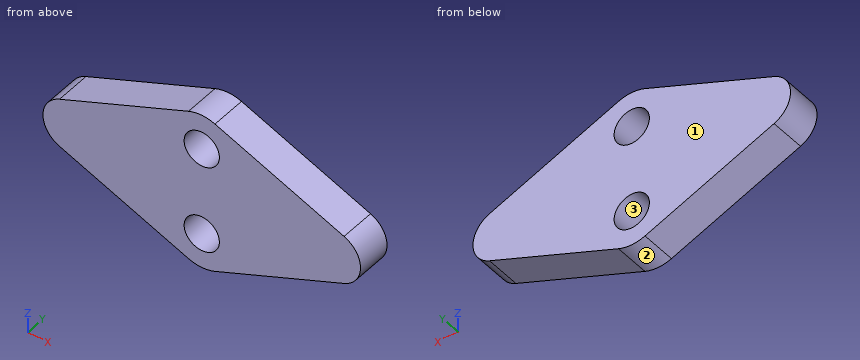
Autodesk Inventor part; units mm, degrees
ref_plane "YZ Plane" through (0, 0, 0) normal (1, 0, 0) x (0, 1, 0)
ref_plane "XZ Plane" through (0, 0, 0) normal (0, 1, 0) x (-1, 0, 0)
ref_plane "XY Plane" through (0, 0, 0) normal (0, 0, 1) x (1, 0, 0)
sketch "スケッチ1" plane through (0, 0, 0) normal (0, 1, 0) x (-1, 0, 0)
  circle A0 centre (7.5, 0) radius 1.5
  circle A1 centre (0, 2.5) radius 2
  circle A2 centre (0, -2.5) radius 2
  circle A3 centre (-7.5, 0) radius 1.5
  line L0 (7.5, 0) -> (-7.5, 0) construction
  line L1 (0, -2.5) -> (0, 2.5) construction
  line L2 (0.7512, 4.3536) -> (8.0634, 1.3902)
  line L3 (8.0634, -1.3902) -> (0.7512, -4.3536)
  line L4 (-0.7512, -4.3536) -> (-8.0634, -1.3902)
  line L5 (-8.0634, 1.3902) -> (-0.7512, 4.3536)
  point P0 (0, 0)
  point P1 (0, 0)
  dimension "d0" = 5
  dimension "d1" = 15
  dimension "d2" = 4
  dimension "d3" = 3
extrude "押し出し1" add sketch "スケッチ1" along normal blind 2
sketch "スケッチ2" plane through (0, 2, 0) normal (0, 1, 0) x (1, 0, 0)
  arc A0 (-0.7512, -4.3536) -> (0.7512, -4.3536) centre (0, -2.5) ccw
  arc A1 (0.7512, 4.3536) -> (-0.7512, 4.3536) centre (0, 2.5) ccw
  point P0 (0, 0)
hole "穴1" at (0, 2, 2.5) at (0, 2, -2.5) direction (0, -1, 0) diameter 2 end through all
properties part number "Band_Cap"
Build history of the part. All positions in model axes, mm. Face numbers are marked on the shaded views. Round coordinates to 2 decimals unless told otherwise and drop trailing zeros. Loops run counter-clockwise (first coordinate to the right, second up) from the corner with the lowest first, then second, coordinate; pieces in that order, holes last. Notation, with made-up numbers: (30.5, 59) -> (50.5, 59) arc R26 cw to (50.5, 74) -> close; hole circle Ø1 at (21, 30.5). An arc over 180 degrees is marked (long way). Use CSV: the item, a comma, the result in double quotes. Start each with the question number.
Q1. Saw through at A-A on z = -2.5. Give the cut face in (x, y), and give its area (3 significant figures).
Q2. Drill centre lines: L1, parallel to Z at x = 0.75, y = 0.9; L2, parallel to X at y = 0.65, z = -2.5; L3, parallel to X at y = 0.8, z = -1.75. Where is each one in solid material? Low to high.
Q3. Saw through at B-B on y = 1.3. Give the cut face in (x, z).
Q4. Saw through at C-C on x = -7.25. Give the cut face in (y, z).
Q5. Flat gauge pin, fed straight in: pin 1 Ø1.8 at (x, z) = (0, -2.5) entering from -Y. Where does the tip first touch, or does it go through?
Q6. Saw through at D-D on z = 3.25. Give the cut face in (x, y), and give its area (3 significant figures).
Q7. Mould opens along X. For the marked faces 1, 2 and 3 say: +X half, -X half, draft (parallel to the pull), parting line (faces both ways), or undercut.
Solutions:
1,outline,"(-5.32, 0) -> (-1, 0) -> (-1, 2) -> (-5.32, 2) -> close; (1, 0) -> (5.32, 0) -> (5.32, 2) -> (1, 2) -> close"
1,area,"17.3 mm^2"
2,L1,"z = -4.35 to -3.16, -1.84 to 1.84, 3.16 to 4.35"
2,L2,"x = -5.32 to -1, 1 to 5.32"
2,L3,"x = -7.18 to -0.66, 0.66 to 7.18"
3,outline,"(-8.06, -1.39) -> (-0.75, -4.35) arc R2 ccw to (0.75, -4.35) -> (8.06, -1.39) arc R1.5 ccw to (8.06, 1.39) -> (0.75, 4.35) arc R2 ccw to (-0.75, 4.35) -> (-8.06, 1.39) arc R1.5 ccw to start; hole circle Ø2 at (0, -2.5); hole circle Ø2 at (0, 2.5)"
4,outline,"(0, -1.72) -> (2, -1.72) -> (2, 1.72) -> (0, 1.72) -> close"
5,pin 1,"passes through"
6,outline,"(-3.47, 0) -> (-0.66, 0) -> (-0.66, 2) -> (-3.47, 2) -> close; (0.66, 0) -> (3.47, 0) -> (3.47, 2) -> (0.66, 2) -> close"
6,area,"11.3 mm^2"
7,face 1,"draft"
7,face 2,"parting line"
7,face 3,"undercut"
